The figure shows three views and two pictorial views of one solid part (mm, origin at its lowest corner). Answer the questions. A direction names the side the tool comes from. Round coordinates to 2 decimals unless told otherwise and drop trailing zeros. Order: outer loops, then holes, each group sorted by start corner. A loop starts at its lowest first (then second) coordinate and runs counter-clockwise, first axis right, second up. Notation, with made-up numbers: (45, -37) -> (70, -37) arc R25 cw to (70, -8) -> close; hole circle Ø11 at (19, 13). An arc over 180 degrees is marked (long way). Return JSON: item names as keys, results as strings. Group by question number.
(1) The part is cut by section D-D (x = 6). Determine the outline of the cut face in (y, z) (1 decimal), plus the area to 3 significant figures.
(2) The part is cut by section C-C (z = 24.5). Determine the outline of the cut face in (x, y).
(3) Consider line 1 (X direction, y = 0.95, z = 14.5); line 2 (Z direction, x = 2, y = 0.5); line 3 (X direction, y = 3.35, z = 14.5) (1 decimal). Determine where each line is inside the solid, lowest interval first. Write a range as [from, to].
(4) Determine the mould class of the marked faces 1, 2 and 3 for opening direction X: +X half, -X half, draft (parallel to the pull), parting line (faces both ways), or undercut.
(5) The part is cut by section B-B (y = 0.45). Count the separate pieces of the cut face and the enclosed holes in it, plus the area to 3 significant figures.
(6) The part is cut by section A-A (z = 14.5). Determine the outline of the cut face in (x, y) (1 decimal).
(7) Which of the six approach directions +Z, -Z, +X, -X, +Y, -Y give full straight-line access (tool end or side, diameter ignored) to the marked faces 4 and 5?
(8) Each of these flat-tipped pins is pushed along its axis until it touches: pin 1 (1.4 mm diameter, centred on x = 13.5, y = 1, fed in from +Z); pin 2 (1.4 mm diameter, centred on x = 13.5, y = 1, fed in from -Z); pin 3 (1.5 mm diameter, centred on y = 1, z = 15.5, fed in from -X). Where does it stop, or does it pass through?
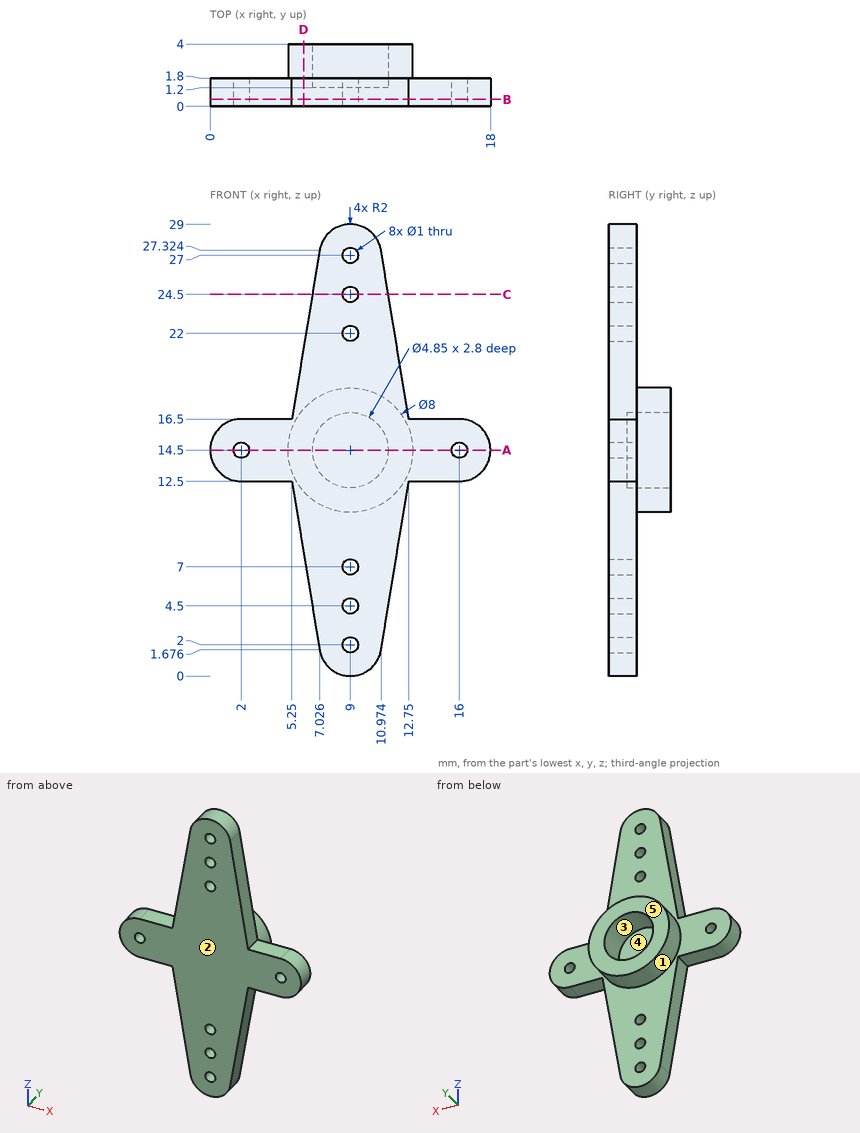
Answer below:
{
 "1": {"outline": "(0, 7.9) -> (1.8, 7.9) -> (1.8, 11.9) -> (4, 11.9) -> (4, 17.1) -> (1.8, 17.1) -> (1.8, 21.1) -> (0, 21.1) -> close", "area": "35.3 mm²"},
 "2": {"outline": "(6.56, 0) -> (8.5, 0) -> (8.5, 1.8) -> (6.56, 1.8) -> close; (9.5, 0) -> (11.44, 0) -> (11.44, 1.8) -> (9.5, 1.8) -> close"},
 "3": {"line 1": "x = [0, 1.5], [2.5, 15.5], [16.5, 18]", "line 2": "z = [12.5, 14], [15, 16.5]", "line 3": "x = [5, 6.6], [11.4, 13]"},
 "4": {"face 1": "parting line", "face 2": "draft", "face 3": "undercut"},
 "5": {"separate pieces": "1", "enclosed holes": "8", "area": "196 mm²"},
 "6": {"outline": "(0, 0) -> (1.5, 0) -> (1.5, 1.8) -> (0, 1.8) -> close; (2.5, 0) -> (15.5, 0) -> (15.5, 1.8) -> (13, 1.8) -> (13, 4) -> (11.4, 4) -> (11.4, 1.2) -> (6.6, 1.2) -> (6.6, 4) -> (5, 4) -> (5, 1.8) -> (2.5, 1.8) -> close; (16.5, 0) -> (18, 0) -> (18, 1.8) -> (16.5, 1.8) -> close"},
 "7": {"face 4": "+Y", "face 5": "+Z, -Z, +X, -X, +Y"},
 "8": {"pin 1": "stops at z = 16.5", "pin 2": "stops at z = 12.5", "pin 3": "stops at x = 0.02"}
}
